from build123d import *

# Parameters (mm, degrees)
SKETCH1_W           = 127
SKETCH1_H           = 50.8
BOSS_EXTRUDE1_DEPTH = 25.4
SKETCH2_R           = 15.875
CUT_EXTRUDE1_DEPTH  = 26.4


with BuildPart() as part:
    # Sketch1 → Boss-Extrude1 (new body)
    with BuildSketch(Plane(origin=(0, 0, 0), x_dir=(1, 0, 0), z_dir=(0, 1, 0))):
        with Locations((63.5, 25.4)):
            Rectangle(SKETCH1_W, SKETCH1_H)
    extrude(amount=BOSS_EXTRUDE1_DEPTH)

    # Sketch2 → Cut-Extrude1 (cut, through all)
    with BuildSketch(Plane(origin=(0, 25.4, 0), x_dir=(1, 0, 0), z_dir=(0, 1, 0))):
        with Locations((31.75, 25.4)):
            Circle(SKETCH2_R)
        with Locations((95.25, 25.4)):
            Circle(SKETCH2_R)
    extrude(amount=-CUT_EXTRUDE1_DEPTH, mode=Mode.SUBTRACT)


solid = part.part
Model file for the job. Use its own axes, mm. Round coordinates to 2 decimals unless told otherwise and drop trailing zeros. Order: outer loops, then holes, each group sorted by start corner. A loop starts at its lowest first (then second) coordinate and runs counter-clockwise, first axis right, second up.
(1) Band-saw the part on B-B (z = -25.4). List the corners of the cut face in (x, y) (3 decimals), then the cut area to 3 significant figures.
(2) Pin check, flat tip, straight feed: pin 1 (10 mm diameter, centred on x = 80.5, z = -21, fed in from -Y). Stop position of the tip, or through.
(3) Band-saw the part on A-A (x = 95.25). List the corners of the cut face in (y, z) (3 decimals), then the cut area to 3 significant figures.
(4) Band-saw the part on D-D (x = 36). List the corners of the cut face in (y, z).
(5) Band-saw the part on C-C (y = 3.5). List the corners of the cut face in (x, z) (3 decimals), then the cut area to 3 significant figures.
(6) Drill centre lines: line 1 (X direction, y = 14.75, z = -25.4) (3 decimals); line 2 (Z direction, x = 95.25, y = 13) (3 decimals); line 3 (X direction, y = 16, z = -37). Where is each one in solid material? Low to high.
(7) Pull direction X, two halves, no side cores. Call faces 1 (the face through (110.39, 12.88, -30.17)), 2 (the face through (63, 13, -50.8)), 3 (the face through (0, 13, -25)), 4 (the face through (127, 13, -25)): released by +X, released by -X, zero draft, split by the parting line, or undercut.
Verdict:
1. outline: (0, 0) - (15.875, 0) - (15.875, 25.4) - (0, 25.4) - close; (47.625, 0) - (79.375, 0) - (79.375, 25.4) - (47.625, 25.4) - close; (111.125, 0) - (127, 0) - (127, 25.4) - (111.125, 25.4) - close
1. area: 1,610 mm2
2. pin 1: stops at y = 0
3. outline: (0, -50.8) - (25.4, -50.8) - (25.4, -41.275) - (0, -41.275) - close; (0, -9.525) - (25.4, -9.525) - (25.4, 0) - (0, 0) - close
3. area: 484 mm2
4. outline: (0, -50.8) - (25.4, -50.8) - (25.4, -40.7) - (0, -40.7) - close; (0, -10.1) - (25.4, -10.1) - (25.4, 0) - (0, 0) - close
5. outline: (0, -50.8) - (127, -50.8) - (127, 0) - (0, 0) - close; hole circle Ø31.75 at (31.75, -25.4); hole circle Ø31.75 at (95.25, -25.4)
5. area: 4,870 mm2
6. line 1: x = 0 to 15.875, 47.625 to 79.375, 111.125 to 127
6. line 2: z = -50.8 to -41.275, -9.525 to 0
6. line 3: x = 0 to 20.91, 42.59 to 84.41, 106.09 to 127
7. face 1: undercut
7. face 2: zero draft
7. face 3: released by -X
7. face 4: released by +X
